For this review, use the dimensioned drawing (mm, ordinates from the lowest corner) and the shaded views. Coordinates: 2 decimals unless noted, no trailing zeros. Loops run counter-clockwise (first coordinate to the right, second up) from the corner with the lowest first, then second, coordinate; pieces in that order, holes last. Notation, with made-up numbers: M 18.5,35 L 50.5,35 A27 cw 50.5,61 Z; hole C -35.75,-26 d10. An arc over 180 degrees is marked long. One line per item, written item: value.
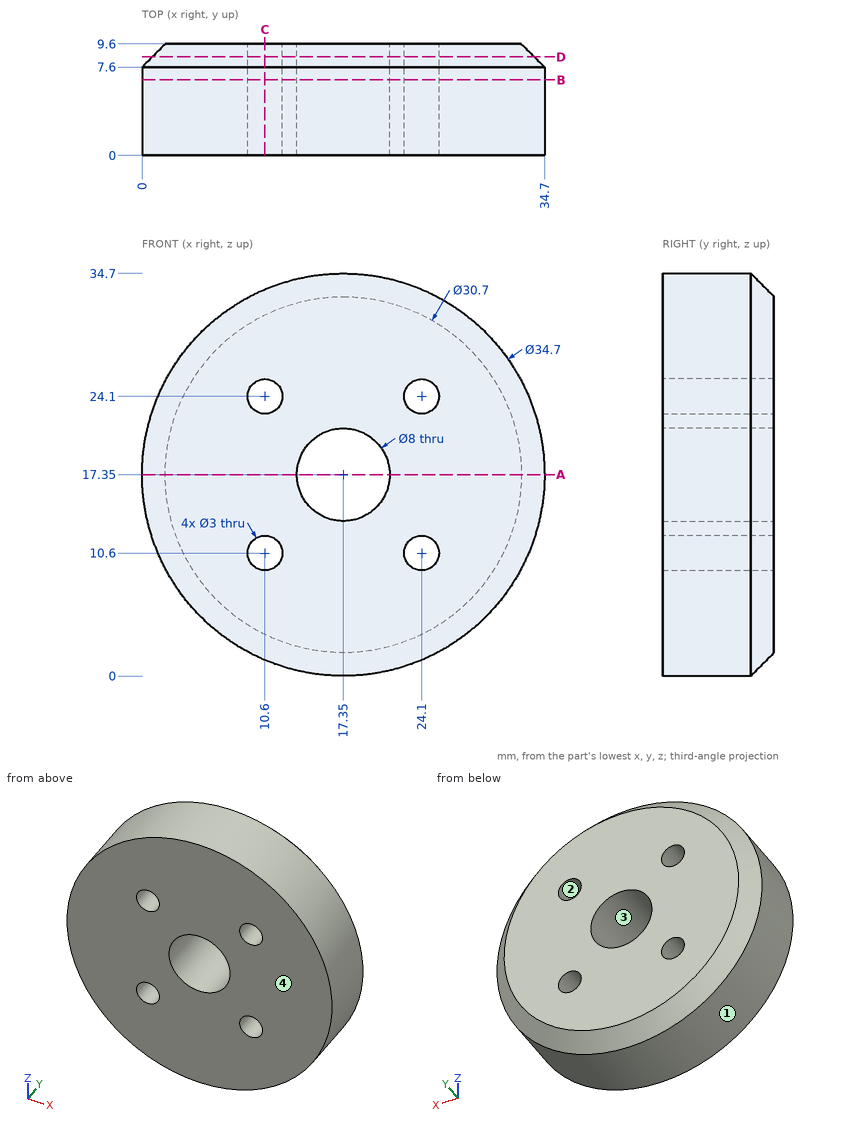
(1) Add section A-A on z = 17.35. State the section outline as (x, y) points, then the cut area to 3 significant figures.
Checks:
outline: M 0,0 L 13.35,0 L 13.35,9.6 L 2,9.6 L 0,7.6 Z; M 21.35,0 L 34.7,0 L 34.7,7.6 L 32.7,9.6 L 21.35,9.6 Z
area: 252 mm^2
(2) Add section C-C on x = 10.6. State how many separate pieces and enclosed holes the cut face has, then the cut area to 3 significant figures.
Checks:
separate pieces: 3
enclosed holes: 0
area: 245 mm^2
(3) Add section B-B on y = 6.5. State the section outline as (x, z) points.
Checks:
outline: C 17.35,17.35 d34.7; hole C 10.6,10.6 d3; hole C 10.6,24.1 d3; hole C 17.35,17.35 d8; hole C 24.1,10.6 d3; hole C 24.1,24.1 d3
(4) To check wall thickness, follow L1, parallel to X at y = 6.75, z = 17.35; L2, parallel to X at y = 4.25, z = 24.1; L3, parallel to X at y = 1.75, z = 24.5. State the ranges of each line that lie inside material, in increasing order. Write a range as [from, to].
Checks:
L1: [0, 13.35], [21.35, 34.7]
L2: [1.37, 9.1], [12.1, 22.6], [25.6, 33.33]
L3: [1.54, 9.15], [12.05, 22.65], [25.55, 33.16]
(5) Draft analysis for pull direction X (two halves, no side actions). For the marked faces 1, 2, 3 and 4, state which applies: pulls with the +X half, pulls with the -X half, needs draft (parallel to the pull), parting line crosses it, or undercut.
Checks:
face 1: parting line crosses it
face 2: undercut
face 3: undercut
face 4: needs draft
(6) Add section D-D on y = 8.5. State the section outline as (x, z) points.
Checks:
outline: C 17.35,17.35 d32.9; hole C 10.6,10.6 d3; hole C 10.6,24.1 d3; hole C 17.35,17.35 d8; hole C 24.1,10.6 d3; hole C 24.1,24.1 d3
(7) Insertion check: pin 1 Ø4 at (x, z) = (20.5, 12.5) entering from -Y; pin 2 Ø5 at (y, z) = (2.5, 11) entering from +X; pin 3 Ø1 at (y, z) = (3.5, 6) entering from +X; pin 4 Ø3 at (y, z) = (7, 27) entering from -X. Each pin has a flat end and moves straight along its axis. Give the tip position at first contact, or say it passes through.
Checks:
pin 1: y = 0
pin 2: x = 34.27
pin 3: x = 30.89
pin 4: x = 2.03
